Part model, mm, in its own coordinate system. A direction names the side the tool comes from. Give positions to 0.01 mm unless a question says otherwise; leave off trailing zeros. Loops run counter-clockwise (first coordinate to the right, second up) from the corner with the lowest first, then second, coordinate; pieces in that order, holes last. Notation, with made-up numbers: (-30.5, 52) -> (1.5, 52) arc R32 ccw to (1.5, 85) -> close; hole circle Ø3 at (88.25, 77). An arc over 180 degrees is marked (long way). One line per question, with ' | ' between items.
```python
from build123d import *

# Parameters (mm, degrees)
SKETCH1_R           = 2.38125
BOSS_EXTRUDE1_DEPTH = 3.175


with BuildPart() as part:
    # Sketch1 → Boss-Extrude1 (new body)
    with BuildSketch(Plane.XY):
        with BuildLine():
            Line((-174.625, 0), (-193.675, 0))
            ThreePointArc((-193.675, 0), (-198.165128061, 1.859871939), (-200.025, 6.35))
            Line((-200.025, 6.35), (-200.025, 28.027709878))
            ThreePointArc((-200.025, 28.027709878), (-198.486650336, 32.171442621), (-194.616961876, 34.307455719))
            Line((-194.616961876, 34.307455719), (-150.166961876, 40.974955719))
            ThreePointArc((-150.166961876, 40.974955719), (-145.081267257, 39.506860214), (-142.875, 34.695209878))
            Line((-142.875, 34.695209878), (-142.875, 6.35))
            ThreePointArc((-142.875, 6.35), (-144.734871939, 1.859871939), (-149.225, 0))
            Line((-149.225, 0), (-161.925, 0))
            Line((-161.925, 0), (-161.925, 3.175))
            Line((-161.925, 3.175), (-174.625, 3.175))
            Line((-174.625, 3.175), (-174.625, 0))
        make_face()
        with Locations((-190.5, 17.4625)):
            Circle(SKETCH1_R, mode=Mode.SUBTRACT)
        with Locations((-152.4, 20.32)):
            Circle(SKETCH1_R, mode=Mode.SUBTRACT)
    extrude(amount=BOSS_EXTRUDE1_DEPTH)


solid = part.part
```
1) Pin check, flat tip, straight feed: P1, Ø1, axis at x = -168.5, z = 2.5, coming from the -Y side (3 decimals). Stop position of the tip, or through.
Found:
P1: y = 3.175
2) Pull direction X, two halves, no side cores. Call faces 3 (the flat face through (-161.925, 2, 2)), 4 (the flat face through (-155, 0, 2)), 5 (the flat face through (-172.703, 37.595, 1.565)): pulls with the +X half, pulls with the -X half, needs draft (parallel to the pull), parting line crosses it, or undercut.
Found:
face 3: undercut | face 4: needs draft | face 5: pulls with the -X half
3) Saw through at A-A (x = -152.4). Give the cut face in (y, z) (3 decimals).
Found:
outline: (0, 0) -> (17.939, 0) -> (17.939, 3.175) -> (0, 3.175) -> close; (22.701, 0) -> (40.64, 0) -> (40.64, 3.175) -> (22.701, 3.175) -> close
4) Saw through at C-C (z = 2). State how many separate pieces and enclosed holes the cut face has, and give its area (3 significant figures).
Found:
separate pieces: 1 | enclosed holes: 2 | area: 2,050 mm2
5) Saw through at B-B (y = 22). Give the cut face in (x, z) (3 decimals).
Found:
outline: (-200.025, 0) -> (-154.088, 0) -> (-154.088, 3.175) -> (-200.025, 3.175) -> close; (-150.712, 0) -> (-142.875, 0) -> (-142.875, 3.175) -> (-150.712, 3.175) -> close
6) Saw through at D-D (x = -176.5). Give the cut face in (y, z) (3 decimals).
Found:
outline: (0, 0) -> (37.025, 0) -> (37.025, 3.175) -> (0, 3.175) -> close
7) Drill centre lines: line 1 (X direction, y = 20.5, z = 1.75) (3 decimals); line 2 (Y direction, x = -152.4, z = 0.8); line 3 (Y direction, x = -152, z = 2.1). Where is each one in solid material? Low to high.
Found:
line 1: -200.025 to -154.774, -150.026 to -142.875 | line 2: 0 to 17.94, 22.7 to 40.64 | line 3: 0 to 17.97, 22.67 to 40.7
8) Tool access for faces 1 (the flat face through (-174.625, 2, 2)), 2 (the cylindrical face through (-192.88, 17.57, 1.57)): list every direction of +Z, -Z, +X, -X, +Y, -Y with a clear straight run to the whole face (end or side of a thin tool).
Found:
face 1: +Z, -Z, -Y | face 2: +Z, -Z
